```python
from build123d import *

# Parameters (mm, degrees)
BOSS_EXTRUDE1_DEPTH = 0.75
SKETCH2_R           = 1.584525309
SKETCH2_R_2         = 0.75
CUT_EXTRUDE1_DEPTH  = 2
CUT_EXTRUDE2_START  = -2
SKETCH3_R           = 1.564549905
SKETCH3_R_2         = 0.75
CUT_EXTRUDE2_DEPTH  = 2


with BuildPart() as part:
    # Sketch1 → Boss-Extrude1 (new body)
    with BuildSketch(Plane.XY):
        Polygon((12, 0), (-12, 0), (-12, 1.5), (-10, 1.5), (-10, 9.5), (-12.8, 9.5), (-12.8, 27.5), (12.8, 27.5), (12.8, 9.5), (10, 9.5), (10, 1.5), (12, 1.5), align=None)
    extrude(amount=BOSS_EXTRUDE1_DEPTH)

    # Sketch2 → Cut-Extrude1 (cut)
    with BuildSketch(Plane.ZY.offset(12)):
        with Locations((0.375, 0.75)):
            Circle(SKETCH2_R)
        with Locations((0.375, 0.75)):
            Circle(SKETCH2_R_2, mode=Mode.SUBTRACT)
    extrude(amount=-CUT_EXTRUDE1_DEPTH, mode=Mode.SUBTRACT)

    # Sketch3 → Cut-Extrude2 (cut)
    with BuildSketch(Plane(origin=(12, 0, 0), x_dir=(0, 0, -1), z_dir=(1, 0, 0)).offset(CUT_EXTRUDE2_START)):
        with Locations((-0.375, 0.75)):
            Circle(SKETCH3_R)
        with Locations((-0.375, 0.75)):
            Circle(SKETCH3_R_2, mode=Mode.SUBTRACT)
    extrude(amount=CUT_EXTRUDE2_DEPTH, mode=Mode.SUBTRACT)


solid = part.part
```
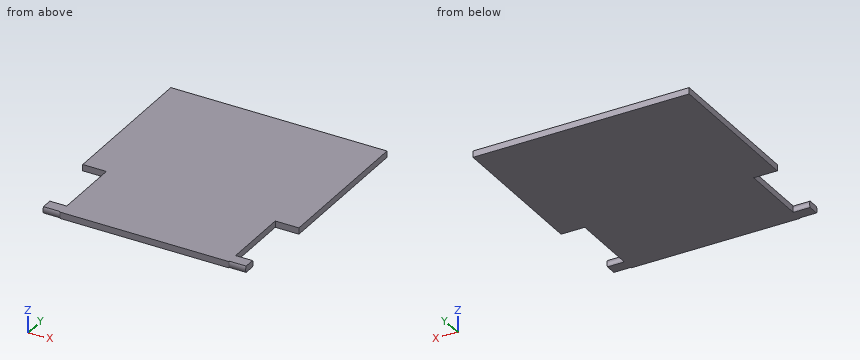
Input: part model. Units: mm. Frame: model coordinates. Coordinates: 2 decimals unless noted, no trailing zeros. Write each loop counter-clockwise with the first axis right and the second up, starting at its lowest first coordinate (ties: lowest second). Pieces come first, ordered by that corner, then holes. Notation, with made-up numbers: M 33,-19.75 L 59,-19.75 A18 ccw 59,9.25 Z; hole C 52,71.25 d1. An arc over 180 degrees is marked long. Use one line per item in the form item = value.
Q1. Material intervals for probe 1 along Y at (x, z) = (10.5, 0.45); probe 2 along X at (y, z) = (5, 0.5); probe 3 along X at (y, z) = (1.25, 0.4), sorted ascending. Write a range as from..to.
Answer below:
probe_1 = 0..1.5, 9.5..27.5
probe_2 = -10..10
probe_3 = -12..12
Q2. Section C-C (y = 7). Return loops of the section in (x, z).
Answer below:
outline = M -10,0 L 10,0 L 10,0.75 L -10,0.75 Z
Q3. Section A-A (x = 10.75). Return loops of the section in (y, z) (3 decimals).
Answer below:
outline = M 0.1,0 L 1.4,0 A0.75 ccw 1.4,0.75 L 0.1,0.75 A0.75 ccw Z; M 9.5,0 L 27.5,0 L 27.5,0.75 L 9.5,0.75 Z
